Geometry: final body of the model. Coordinates: model frame, mm. A direction names the side the tool comes from. Give positions to 0.01 mm unless a question says otherwise; leave off trailing zeros. Write each loop counter-clockwise with the first axis right and the second up, starting at its lowest first coordinate (ties: lowest second). Pieces come first, ordered by that corner, then holes. Notation, with made-up numbers: (18.5, 10) -> (73.5, 10) arc R18 ccw to (73.5, 20) -> close; hole circle Ø11 at (74, 59). An arc over 180 degrees is marked (long way). Answer in a Markdown table with one row per item. Add a question column.
Item 1: Access query for faces 4 (the flat face through (13.25, 51.5, 64.58)), 5 (the flat face through (-9.5, 51.5, 65.9)), 6 (the flat face through (-3.7, 46, 66)), 7 (the flat face through (11, 55.4, 66)). Directions: +Z, -Z, +X, -X, +Y, -Y. A direction counts if a zero-diameter tool reaches every point of the face in a straight line with its end or side. Return the directions, or none.
Item 2: First-contact query: P1, Ø6, axis at x = 9, y = 47, coming from the +Z side; P2, Ø1.3, axis at y = 57.5, z = 64, coming from the +X side; P3, Ø6, axis at y = 34, z = 67.5, coming from the -X side; P4, Ø5, axis at y = 37, z = 68.5, coming from the +X side. Flat tips, straight axial feed; report the tip coordinate or a pass-through.
Item 3: Draft query along Z for faces 1 (the flat face through (6.9, 39, 66)), 2 (the flat face through (0, 46, 64.4)), 3 (the flat face through (17.25, 53.48, 62.05)). Return one class per face: +Z half, -Z half, draft (parallel to the pull), parting line (faces both ways), or undercut.
Item 4: Section query A-A on y = 40. Output: boundary loops of the cut face in (x, z), plus the area to 3 significant figures.
Item 5: Section query B-B on z = 66. Output: boundary loops of the cut face in (x, y), plus the area to 3 significant figures.
Item 6: Material intervals for probe 1 along X at (y, z) = (61.7, 66); probe 2 along Y at (x, z) = (0, 61.7); probe 3 along X at (y, z) = (40, 70.15), sorted ascending. Write a range as from..to.
Item 7: Section query D-D on y = 54. Output: boundary loops of the cut face in (x, z).
Item 8: Section query C-C on x = 0. Output: boundary loops of the cut face in (y, z).
```python
from build123d import *

# Parameters (mm, degrees)
CUBE022_W                = 7.4
CUBE022_H                = 50
CUBE022_DEPTH            = 3.2
CUBE023_W                = 15
CUBE023_H                = 4.2
CUBE023_DEPTH            = 12
CYLINDER014_R            = 2.1
CYLINDER014_DEPTH        = 13
PRISM016_DEPTH           = 13
PRISM016_ROLL_ANGLE      = 90
PRISM016_PITCH_ANGLE     = 65.000022
PRISM017_DEPTH           = 13
PRISM017_ROLL_ANGLE      = -90
PRISM017_PITCH_ANGLE     = 4.999997
PRISM017_PLACEMENT_ANGLE = 180
CYLINDER013_R            = 2.3
CYLINDER013_DEPTH        = 41
PRISM014_DEPTH           = 12
PRISM014_PLACEMENT_ANGLE = 15
PRISM015_DEPTH           = 12
PRISM015_PLACEMENT_ANGLE = 75
CUBE021_W                = 30
CUBE021_H                = 12
CUBE021_DEPTH            = 12
CUBE020_W                = 13.8
CUBE020_H                = 23
CUBE020_DEPTH            = 12


with BuildPart() as cube022:
    # cube022 → cube022 (new body)
    with BuildSketch(Plane(origin=(-3.7, 15, 64.4), x_dir=(1, 0, 0), z_dir=(0, 0, 1))):
        with Locations((3.7, 25)):
            Rectangle(CUBE022_W, CUBE022_H)
    extrude(amount=CUBE022_DEPTH)


with BuildPart() as cube023:
    # cube023 → cube023 (new body)
    with BuildSketch(Plane(origin=(5.1, 55.4, 60), x_dir=(1, 0, 0), z_dir=(0, 0, 1))):
        with Locations((7.5, 2.1)):
            Rectangle(CUBE023_W, CUBE023_H)
    extrude(amount=CUBE023_DEPTH)


with BuildPart() as cylinder014:
    # cylinder014 → cylinder014 (new body)
    with BuildSketch(Plane(origin=(15, 64, 66), x_dir=(1, 0, 0), z_dir=(0, -1, 0))):
        Circle(CYLINDER014_R)
    extrude(amount=CYLINDER014_DEPTH)


with BuildPart() as prism016:
    # prism016 → prism016 (new body)
    with BuildSketch(Plane.XY):
        Polygon((5.25, 0), (-2.625, 4.546633), (-2.625, -4.546633), align=None)
    extrude(amount=PRISM016_DEPTH)


with BuildPart() as prism016_1:
    # prism016 roll: moved
    add(prism016.part.rotate(Axis((0, 0, 0), (1, 0, 0)), PRISM016_ROLL_ANGLE))


with BuildPart() as prism016_2:
    # prism016 pitch: moved
    add(prism016_1.part.rotate(Axis((0, 0, 0), (0, 1, 0)), PRISM016_PITCH_ANGLE))


with BuildPart() as prism016_3:
    # prism016 placement: moved
    add(prism016_2.part.moved(Location((18.9, 64, 72))))


with BuildPart() as prism017:
    # prism017 → prism017 (new body)
    with BuildSketch(Plane.XY):
        Polygon((5.25, 0), (-2.625, 4.546633), (-2.625, -4.546633), align=None)
    extrude(amount=PRISM017_DEPTH)


with BuildPart() as prism017_1:
    # prism017 roll: moved
    add(prism017.part.rotate(Axis((0, 0, 0), (1, 0, 0)), PRISM017_ROLL_ANGLE))


with BuildPart() as prism017_2:
    # prism017 pitch: moved
    add(prism017_1.part.rotate(Axis((0, 0, 0), (0, 1, 0)), PRISM017_PITCH_ANGLE))


with BuildPart() as prism017_3:
    # prism017 placement: moved
    add(prism017_2.part.moved(Location((18.9, 64.000001, 60))).rotate(Axis((18.9, 64.000001, 60), (0, 0, 1)), PRISM017_PLACEMENT_ANGLE))


with BuildPart() as group009:
    # cylinder013 → cylinder013 (new body)
    with BuildSketch(Plane(origin=(0, 40, 51.5), x_dir=(1, 0, 0), z_dir=(0, 0, 1))):
        Circle(CYLINDER013_R)
    extrude(amount=CYLINDER013_DEPTH)

    # Group009: union cube022, cube023, cylinder014, prism016, prism017
    add(cube022.part)
    add(cube023.part)
    add(cylinder014.part)
    add(prism016_3.part)
    add(prism017_3.part)


with BuildPart() as prism014:
    # prism014 → prism014 (new body)
    with BuildSketch(Plane.XY):
        Polygon((3, 0), (-1.5, 2.598076), (-1.5, -2.598076), align=None)
    extrude(amount=PRISM014_DEPTH)


with BuildPart() as prism014_1:
    # prism014 placement: moved
    add(prism014.part.moved(Location((7, 51.6, 60))).rotate(Axis((7, 51.6, 60), (0, 0, 1)), PRISM014_PLACEMENT_ANGLE))


with BuildPart() as prism015:
    # prism015 → prism015 (new body)
    with BuildSketch(Plane.XY):
        Polygon((3, 0), (-1.5, 2.598076), (-1.5, -2.598076), align=None)
    extrude(amount=PRISM015_DEPTH)


with BuildPart() as prism015_1:
    # prism015 placement: moved
    add(prism015.part.moved(Location((-7, 51.6, 60))).rotate(Axis((-7, 51.6, 60), (0, 0, -1)), PRISM015_PLACEMENT_ANGLE))


with BuildPart() as cube021:
    # cube021 → cube021 (new body)
    with BuildSketch(Plane(origin=(-9.9, 51.5, 60), x_dir=(1, 0, 0), z_dir=(0, 0, 1))):
        with Locations((15, 6)):
            Rectangle(CUBE021_W, CUBE021_H)
    extrude(amount=CUBE021_DEPTH)


with BuildPart() as obj1:
    # cube020 → cube020 (new body)
    with BuildSketch(Plane(origin=(-6.9, 28.5, 60), x_dir=(1, 0, 0), z_dir=(0, 0, 1))):
        with Locations((6.9, 11.5)):
            Rectangle(CUBE020_W, CUBE020_H)
    extrude(amount=CUBE020_DEPTH)

    # Group008: union prism014, prism015, cube021
    add(prism014_1.part)
    add(prism015_1.part)
    add(cube021.part)

    # difference005: cut Group009
    add(group009.part, mode=Mode.SUBTRACT)


solid = obj1.part
```
Findings below:
| question | item | result |
|---|---|---|
| 1 | face 4 | +Z, -Z, +X, -Y |
| 1 | face 5 | +Z, -Z, -X, -Y |
| 1 | face 6 | +Y, -Y |
| 1 | face 7 | +Z, -Z, +X |
| 2 | P1 | stops at z = 72 |
| 2 | P2 | stops at x = 5.1 |
| 2 | P3 | stops at x = -6.9 |
| 2 | P4 | stops at x = 6.9 |
| 3 | face 1 | draft |
| 3 | face 2 | undercut |
| 3 | face 3 | -Z half |
| 4 | outline | (-6.9, 60) -> (-2.3, 60) -> (-2.3, 64.4) -> (-3.7, 64.4) -> (-3.7, 67.6) -> (-2.3, 67.6) -> (-2.3, 72) -> (-6.9, 72) -> close; (2.3, 60) -> (6.9, 60) -> (6.9, 72) -> (2.3, 72) -> (2.3, 67.6) -> (3.7, 67.6) -> (3.7, 64.4) -> (2.3, 64.4) -> close |
| 4 | area | 101 mm^2 |
| 5 | outline | (-9.9, 51.5) -> (-9.02, 51.5) -> (-6.9, 49.38) -> (-6.9, 28.5) -> (-3.7, 28.5) -> (-3.7, 63.5) -> (-9.9, 63.5) -> close; (3.7, 28.5) -> (6.9, 28.5) -> (6.9, 49.38) -> (9.02, 51.5) -> (12.9, 51.5) -> (12.9, 55.4) -> (5.1, 55.4) -> (5.1, 59.6) -> (12.9, 59.6) -> (12.9, 63.5) -> (3.7, 63.5) -> close; (17.1, 51.5) -> (20.1, 51.5) -> (20.1, 55.4) -> (17.1, 55.4) -> close; (17.1, 59.6) -> (20.1, 59.6) -> (20.1, 63.5) -> (17.1, 63.5) -> close |
| 5 | area | 327 mm^2 |
| 6 | probe 1 | x = -9.9..-3.7, 3.7..12.9, 17.1..20.1 |
| 6 | probe 2 | y = 28.5..37.7, 42.3..63.5 |
| 6 | probe 3 | x = -6.9..-2.3, 2.3..6.9 |
| 7 | outline | (-9.9, 60) -> (14.32, 60) -> (20.1, 64.04) -> (20.1, 67.96) -> (14.32, 72) -> (-9.9, 72) -> close; hole (-3.7, 64.4) -> (3.7, 64.4) -> (3.7, 67.6) -> (-3.7, 67.6) -> close; hole circle Ø4.2 at (15, 66) |
| 8 | outline | (28.5, 60) -> (37.7, 60) -> (37.7, 64.4) -> (28.5, 64.4) -> close; (28.5, 67.6) -> (37.7, 67.6) -> (37.7, 72) -> (28.5, 72) -> close; (42.3, 60) -> (63.5, 60) -> (63.5, 64.4) -> (42.3, 64.4) -> close; (42.3, 67.6) -> (63.5, 67.6) -> (63.5, 72) -> (42.3, 72) -> close |
